Check sheet for the modelled part. Datum: model origin and axes. Units: mm. A direction names the side the tool comes from. Round coordinates to 2 decimals unless told otherwise and drop trailing zeros. Loops run counter-clockwise (first coordinate to the right, second up) from the corner with the lowest first, then second, coordinate; pieces in that order, holes last. Notation, with made-up numbers: M -35.75,13.5 L 13.25,13.5 A6 cw 13.25,23.5 Z; hole C 0,-39.75 d4. An arc over 180 degrees is marked long. One line per question, with ' | ' between items. Start each with the question number.
(1) Section check A-A (x = 4). Record the boundary of the cut face in (y, z), and give its area (3 significant figures).
(2) Section check D-D (y = -14). Record the boundary of the cut face in (x, z), and give its area (3 significant figures).
(3) Section check B-B (y = 4.5). Record the boundary of the cut face in (x, z).
(4) Tool access check on faces 5 (the face through (18.5, -0.2, -0.5)), 6 (the face through (15, -13, -0.5)), 7 (the face through (-15, 13, -0.5)), 8 (the face through (7.5, -12.4, 14.5)), 9 (the face through (-7.5, -12.4, 14.5)). Record the directions out of +Z, -Z, +X, -X, +Y, -Y that give a thin tool (end or side, any length) a straight path to the whole face; none if there is none.
(5) Section check C-C (z = 11.5). Record the boundary of the cut face in (x, y).
(6) Thickness scan on probe 1 along Z at (x, y) = (11, -11); probe 2 along Z at (x, y) = (-12, 4.5); probe 3 along Y at (x, z) = (-3, 19). Record the ranges inside material, lowest first. Write a range as [from, to].
(7) Draft check along X on faces 1 (the face through (0, 0, 7)), 2 (the face through (-18.5, -0.2, -0.5)), 3 (the face through (0, 0, 0)), 4 (the face through (11.5, -0.2, -0.5)). Enter one of: +X half, -X half, draft (parallel to the pull), parting line (faces both ways), or undercut.
(8) Go/stop test with flat-tipped pins: P1, Ø5, axis at x = 17.5, y = 13, coming from the +Z side; P2, Ø0.5, axis at x = 14, z = -0.5, coming from the +Y side; P3, Ø0.5, axis at y = 6, z = -0.5, coming from the +X side; P4, Ø8.5, axis at y = -6.5, z = 15.5, coming from the -X side. Record where each tip stops, or that it passes through.
```python
from build123d import *

# Parameters (mm, degrees)
SKETCH_1_W      = 44
SKETCH_1_H      = 34
EXTRUDE_1_DEPTH = 5
SKETCH_2_W      = 7
SKETCH_2_H      = 26
EXTRUDE_2_DEPTH = 1
SKETCH_3_W      = 15
SKETCH_3_H      = 17
EXTRUDE_3_DEPTH = 5
SKETCH_4_W      = 15
SKETCH_4_H      = 5
EXTRUDE_4_DEPTH = 20


with BuildPart() as part:
    # 스케치1 → 보스-돌출1 (new body)
    with BuildSketch(Plane.XY):
        Rectangle(SKETCH_1_W, SKETCH_1_H)
    extrude(amount=EXTRUDE_1_DEPTH)

    # 스케치2 → 보스-돌출2 (add)
    with BuildSketch(Plane(origin=(0, 0, 0), x_dir=(-1, 0, 0), z_dir=(0, 0, -1))):
        with Locations((-15, 0)):
            Rectangle(SKETCH_2_W, SKETCH_2_H)
    extrude_2 = extrude(amount=EXTRUDE_2_DEPTH)

    # 대칭 복사1: 보스-돌출2 across plane
    add(extrude_2.mirror(Plane(origin=(0, 0, 0), x_dir=(0, 0, 1), z_dir=(1, 0, 0))))

    # 스케치3 → 보스-돌출3 (add)
    with BuildSketch(Plane.XY.offset(5)):
        with Locations((0, -8.5)):
            Rectangle(SKETCH_3_W, SKETCH_3_H)
    extrude(amount=EXTRUDE_3_DEPTH)

    # 스케치4 → 보스-돌출4 (add)
    with BuildSketch(Plane.XY.offset(10)):
        with Locations((0, -14.5)):
            Rectangle(SKETCH_4_W, SKETCH_4_H)
    extrude(amount=EXTRUDE_4_DEPTH)


solid = part.part
```
The answers:
1) outline: M -17,0 L 17,0 L 17,5 L 0,5 L 0,10 L -12,10 L -12,30 L -17,30 Z | area: 355 mm²
2) outline: M -22,0 L 22,0 L 22,5 L 7.5,5 L 7.5,30 L -7.5,30 L -7.5,5 L -22,5 Z | area: 595 mm²
3) outline: M -22,0 L -18.5,0 L -18.5,-1 L -11.5,-1 L -11.5,0 L 11.5,0 L 11.5,-1 L 18.5,-1 L 18.5,0 L 22,0 L 22,5 L -22,5 Z
4) face 5: -Z, +X, +Y, -Y | face 6: -Z, +X, -X, -Y | face 7: -Z, +X, -X, +Y | face 8: +Z, +X, +Y, -Y | face 9: +Z, -X, +Y, -Y
5) outline: M -7.5,-17 L 7.5,-17 L 7.5,-12 L -7.5,-12 Z
6) probe 1: [0, 5] | probe 2: [-1, 5] | probe 3: [-17, -12]
7) face 1: draft | face 2: -X half | face 3: undercut | face 4: undercut
8) P1: z = 5 | P2: y = 13 | P3: x = 18.5 | P4: through
